from build123d import *

# Parameters (mm, degrees)
SKETCH1_W                      = 40.64
SKETCH1_H                      = 2.54
BASE_EXTRUDE_DEPTH             = 5
SKETCH2_W                      = 1.524
SKETCH2_H                      = 0.254
STANDOFF_WIDTH_DEPTH           = 41.966114046
UPPER_START                    = -19.4945
UPPER_CORE_OUTLINE_W           = 3.3528
UPPER_CORE_OUTLINE_H           = 0.889
UPPER_CORE_DEPTH               = 0.889
LEAD_IN_SIZE                   = 0.3937
LEAD_IN_SIZE2                  = 0.469193389
CORE_PATTERN_COUNT             = 16
CORE_PATTERN_PITCH             = 2.54
LEAD_IN_OF_CORE_PATTERN_SIZE2  = 0.469193389
LEAD_IN_OF_CORE_PATTERN_SIZE   = 0.3937
POSITION_CUT_DEPTH             = 21.964620197
SKETCH10_W                     = 0.2794
SKETCH10_H                     = 0.254
STANDOFF_LENGTH_DEPTH          = 22.07970588
STANDOFF_PATTERN_COUNT         = 16
STANDOFF_PATTERN_PITCH         = 2.54
SKETCH11_W                     = 0.635
SKETCH11_H                     = 0.4064
TAIL_DEPTH                     = 3.175
TAIL_FILLETS_R                 = 0.3175
TAIL_PATTERN_COUNT             = 16
TAIL_PATTERN_PITCH             = 2.54
TAIL_FILLETS_OF_TAIL_PATTERN_R = 0.3175
SKETCH12_W                     = 33.02
SKETCH12_H                     = 7.921
CUT_EXTRUDE1_DEPTH             = 22.07970588


# Read off the part's stored shape, not the designer's step: Upper Core
with BuildPart() as part:
    # Sketch1 → Base-Extrude (new body)
    with BuildSketch(Plane(origin=(0, 0, 0), x_dir=(1, 0, 0), z_dir=(0, 1, 0))):
        Rectangle(SKETCH1_W, SKETCH1_H)
    extrude(amount=BASE_EXTRUDE_DEPTH)

    # Sketch2 → Standoff - Width (cut, through all)
    with BuildSketch(Plane.ZY.offset(20.32)):
        with Locations((0, 0.127)):
            Rectangle(SKETCH2_W, SKETCH2_H)
    extrude(amount=-STANDOFF_WIDTH_DEPTH, mode=Mode.SUBTRACT)

    # Upper Core outline → Upper Core (cut)
    with BuildSketch(Plane.YZ.offset(UPPER_START)):
        with Locations((3.3236, 0)):
            Rectangle(UPPER_CORE_OUTLINE_W, UPPER_CORE_OUTLINE_H)
    upper_core = extrude(amount=UPPER_CORE_DEPTH, mode=Mode.SUBTRACT)

    # Lead-in
    lead_in_edges = [part.edges().sort_by_distance(p)[0] for p in [
        (-19.4945, 5, 0),
        (-19.05, 5, 0.4445),
        (-18.6055, 5, 0),
        (-19.05, 5, -0.4445),
    ]]
    lead_in_side = [part.faces().sort_by_distance(p)[0] for p in [
        (0.146976854, 5, 0),
    ]]
    chamfer(lead_in_edges, length=LEAD_IN_SIZE, length2=LEAD_IN_SIZE2, reference=lead_in_side[0])

    # Core Pattern: Upper Core ×16
    with Locations(*[(i * CORE_PATTERN_PITCH, 0, 0) for i in range(1, CORE_PATTERN_COUNT)]):
        add(upper_core, mode=Mode.SUBTRACT)

    # Lead-in of Core Pattern
    lead_in_of_core_pattern_edges = [part.edges().sort_by_distance(p)[0] for p in [
        (-16.9545, 5, 0),
        (-16.51, 5, 0.4445),
        (-16.0655, 5, 0),
        (-16.51, 5, -0.4445),
        (-14.4145, 5, 0),
        (-13.97, 5, 0.4445),
        (-13.5255, 5, 0),
        (-13.97, 5, -0.4445),
        (-11.8745, 5, 0),
        (-11.43, 5, 0.4445),
        (-10.9855, 5, 0),
        (-11.43, 5, -0.4445),
        (-9.3345, 5, 0),
        (-8.89, 5, 0.4445),
        (-8.4455, 5, 0),
        (-8.89, 5, -0.4445),
        (-6.7945, 5, 0),
        (-6.35, 5, 0.4445),
        (-5.9055, 5, 0),
        (-6.35, 5, -0.4445),
        (-4.2545, 5, 0),
        (-3.81, 5, 0.4445),
        (-3.3655, 5, 0),
        (-3.81, 5, -0.4445),
        (-1.7145, 5, 0),
        (-1.27, 5, 0.4445),
        (-0.8255, 5, 0),
        (-1.27, 5, -0.4445),
        (0.8255, 5, 0),
        (1.27, 5, 0.4445),
        (1.7145, 5, 0),
        (1.27, 5, -0.4445),
        (3.3655, 5, 0),
        (3.81, 5, 0.4445),
        (4.2545, 5, 0),
        (3.81, 5, -0.4445),
        (5.9055, 5, 0),
        (6.35, 5, 0.4445),
        (6.7945, 5, 0),
        (6.35, 5, -0.4445),
        (8.4455, 5, 0),
        (8.89, 5, 0.4445),
        (9.3345, 5, 0),
        (8.89, 5, -0.4445),
        (10.9855, 5, 0),
        (11.43, 5, 0.4445),
        (11.8745, 5, 0),
        (11.43, 5, -0.4445),
        (13.5255, 5, 0),
        (13.97, 5, 0.4445),
        (14.4145, 5, 0),
        (13.97, 5, -0.4445),
        (16.0655, 5, 0),
        (16.51, 5, 0.4445),
        (16.9545, 5, 0),
        (16.51, 5, -0.4445),
        (18.6055, 5, 0),
        (19.05, 5, 0.4445),
        (19.4945, 5, 0),
        (19.05, 5, -0.4445),
    ]]
    chamfer(lead_in_of_core_pattern_edges, length=LEAD_IN_OF_CORE_PATTERN_SIZE, length2=LEAD_IN_OF_CORE_PATTERN_SIZE2)

    # Sketch4 → Position Cut (cut, through all)
    with BuildSketch(Plane(origin=(0, 5, 0), x_dir=(-1, 0, 0), z_dir=(0, 1, 0))):
        Polygon((20.32, 1.016), (20.212646968, 1.016), (20.066, 1.27), (20.32, 1.27), align=None)
        Polygon((20.066, -1.27), (20.32, -1.27), (20.32, -1.016), (20.212646968, -1.016), align=None)
        Polygon((17.78, -1.016), (17.887353032, -1.016), (18.034, -1.27), (17.78, -1.27), align=None)
        Polygon((18.034, 1.27), (17.78, 1.27), (17.78, 1.016), (17.887353032, 1.016), align=None)
    position_cut = extrude(amount=-POSITION_CUT_DEPTH, mode=Mode.SUBTRACT)

    # Sketch10 → Standoff - Length (cut, through all)
    with BuildSketch(Plane.XY.offset(1.27)):
        with Locations((-17.9197, 0.127)):
            Rectangle(SKETCH10_W, SKETCH10_H)
        with Locations((-20.1803, 0.127)):
            Rectangle(SKETCH10_W, SKETCH10_H)
    standoff_length = extrude(amount=-STANDOFF_LENGTH_DEPTH, mode=Mode.SUBTRACT)

    # Standoff Pattern: Position Cut, Standoff - Length ×16
    with Locations(*[(i * STANDOFF_PATTERN_PITCH, 0, 0) for i in range(1, STANDOFF_PATTERN_COUNT)]):
        add(position_cut, mode=Mode.SUBTRACT)
        add(standoff_length, mode=Mode.SUBTRACT)

    # Sketch11 → Tail (add)
    with BuildSketch(Plane.XZ.offset(-0.254)):
        with Locations((-19.05, 0)):
            Rectangle(SKETCH11_W, SKETCH11_H)
    tail = extrude(amount=TAIL_DEPTH)

    # Tail Fillets
    tail_fillets_edges = [part.edges().sort_by_distance(p)[0] for p in [
        (-19.3675, -2.921, 0),
        (-18.7325, -2.921, 0),
    ]]
    fillet(tail_fillets_edges, radius=TAIL_FILLETS_R - 0.0001)  # a hair under: the kernel refuses the full size

    # Tail Pattern: Tail ×16
    with Locations(*[(i * TAIL_PATTERN_PITCH, 0, 0) for i in range(1, TAIL_PATTERN_COUNT)]):
        add(tail)

    # Tail Fillets of Tail Pattern
    tail_fillets_of_tail_pattern_edges = [part.edges().sort_by_distance(p)[0] for p in [
        (-16.8275, -2.921, 0),
        (-16.1925, -2.921, 0),
        (-14.2875, -2.921, 0),
        (-13.6525, -2.921, 0),
        (-11.7475, -2.921, 0),
        (-11.1125, -2.921, 0),
        (-9.2075, -2.921, 0),
        (-8.5725, -2.921, 0),
        (-6.6675, -2.921, 0),
        (-6.0325, -2.921, 0),
        (-4.1275, -2.921, 0),
        (-3.4925, -2.921, 0),
        (-1.5875, -2.921, 0),
        (-0.9525, -2.921, 0),
        (0.9525, -2.921, 0),
        (1.5875, -2.921, 0),
        (3.4925, -2.921, 0),
        (4.1275, -2.921, 0),
        (6.0325, -2.921, 0),
        (6.6675, -2.921, 0),
        (8.5725, -2.921, 0),
        (9.2075, -2.921, 0),
        (11.1125, -2.921, 0),
        (11.7475, -2.921, 0),
        (13.6525, -2.921, 0),
        (14.2875, -2.921, 0),
        (16.1925, -2.921, 0),
        (16.8275, -2.921, 0),
        (18.7325, -2.921, 0),
        (19.3675, -2.921, 0),
    ]]
    fillet(tail_fillets_of_tail_pattern_edges, radius=TAIL_FILLETS_OF_TAIL_PATTERN_R - 0.0001)  # a hair under: the kernel refuses the full size

    # Sketch12 → Cut-Extrude1 (cut, through all)
    with BuildSketch(Plane.XY.offset(1.27)):
        with Locations((3.81, 1.0395)):
            Rectangle(SKETCH12_W, SKETCH12_H)
    extrude(amount=-CUT_EXTRUDE1_DEPTH, mode=Mode.SUBTRACT)


solid = part.part
Part model, mm, in its own coordinate system. A direction names the side the tool comes from. Coordinates: 2 decimals unless noted, no trailing zeros. Order: outer loops, then holes, each group sorted by start corner. A loop starts at its lowest first (then second) coordinate and runs counter-clockwise, first axis right, second up.
(1) Probe L1, parallel to X at y = -0.25, z = 0; L2, parallel to X at y = 1.75, z = -0.35; L3, parallel to X at y = 2.5, z = -1.05. List the from-to ranges inside material, lowest first.
Check sheet entries:
L1: x = -19.37 to -18.73, -16.83 to -16.19, -14.29 to -13.65
L2: x = -20.32 to -19.49, -18.61 to -16.95, -16.07 to -14.41, -13.53 to -12.7
L3: x = -20.19 to -17.91, -17.65 to -15.37, -15.11 to -12.83
(2) Slice it at C-C, the plane y = 0.5. Write the cut outline in (x, z), and give its area (3 significant figures).
Check sheet entries:
outline: (-20.32, -1.02) - (-20.21, -1.02) - (-20.07, -1.27) - (-18.03, -1.27) - (-17.89, -1.02) - (-17.67, -1.02) - (-17.53, -1.27) - (-15.49, -1.27) - (-15.35, -1.02) - (-15.13, -1.02) - (-14.99, -1.27) - (-12.95, -1.27) - (-12.81, -1.02) - (-12.7, -1.02) - (-12.7, 1.02) - (-12.81, 1.02) - (-12.95, 1.27) - (-14.99, 1.27) - (-15.13, 1.02) - (-15.35, 1.02) - (-15.49, 1.27) - (-17.53, 1.27) - (-17.67, 1.02) - (-17.89, 1.02) - (-18.03, 1.27) - (-20.07, 1.27) - (-20.21, 1.02) - (-20.32, 1.02) - close
area: 18.8 mm2
(3) Tool access for faces 4 (the face through (-19, 2, 1.27)), 5 (the face through (-14.414, 3, 0)): list every direction of +Z, -Z, +X, -X, +Y, -Y with a clear straight run to the whole face (end or side of a thin tool).
Check sheet entries:
face 4: +Z, +X, -X, +Y, -Y
face 5: +Y
(4) Slice it at D-D, the plane y = 2.5. State how many separate pieces and enclosed holes the cut face has, and give its area (3 significant figures).
Check sheet entries:
separate pieces: 1
enclosed holes: 3
area: 16.4 mm2
(5) Slice it at B-B, the plane z = -0.35. Write the cut outline in (x, y).
Check sheet entries:
outline: (-20.32, 0.25) - (-12.7, 0.25) - (-12.7, 5) - (-13.13, 5) - (-13.53, 4.53) - (-13.53, 1.65) - (-14.41, 1.65) - (-14.41, 4.53) - (-14.81, 5) - (-15.67, 5) - (-16.07, 4.53) - (-16.07, 1.65) - (-16.95, 1.65) - (-16.95, 4.53) - (-17.35, 5) - (-18.21, 5) - (-18.61, 4.53) - (-18.61, 1.65) - (-19.49, 1.65) - (-19.49, 4.53) - (-19.89, 5) - (-20.32, 5) - close
(6) Slice it at A-A, the plane y = -0.5. Write the cut outline in (x, z), and give its area (3 significant figures).
Check sheet entries:
outline: (-19.37, -0.2) - (-18.73, -0.2) - (-18.73, 0.2) - (-19.37, 0.2) - close; (-16.83, -0.2) - (-16.19, -0.2) - (-16.19, 0.2) - (-16.83, 0.2) - close; (-14.29, -0.2) - (-13.65, -0.2) - (-13.65, 0.2) - (-14.29, 0.2) - close
area: 0.774 mm2
(7) Pin check, flat tips, straight feed: pin 1 Ø1 at (y, z) = (-2, -0.5) entering from +X; pin 2 Ø0.5 at (x, y) = (-19, -0.5) entering from +Z; pin 3 Ø1 at (x, y) = (-18.5, -1.5) entering from -Z. Stop position of each tip, or through.
Check sheet entries:
pin 1: stops at x = -13.65
pin 2: stops at z = 0.2
pin 3: stops at z = -0.2
(8) Pull direction X, two halves, no side cores. Call faces 1 (the face through (-12.7, 3, 0)), 2 (the face through (-14, 2, -1.27)), 3 (the face through (-14, 3, 0.444)): pulls with the +X half, pulls with the -X half, needs draft (parallel to the pull), parting line crosses it, or undercut.
Check sheet entries:
face 1: pulls with the +X half
face 2: needs draft
face 3: undercut
